Source: CAD feature listing. Evaluate the final solid. Frame: model axes, mm. Coordinates: 2 decimals unless noted, no trailing zeros. Order: outer loops, then holes, each group sorted by start corner. A loop starts at its lowest first (then second) coordinate and runs counter-clockwise, first axis right, second up. Notation, with made-up numbers: (19, 73) - (62, 73) arc R19 cw to (62, 107) - close; hole circle Ø2 at (-8, 23.5). An arc over 180 degrees is marked (long way). One line per question, with ' | ' between items.
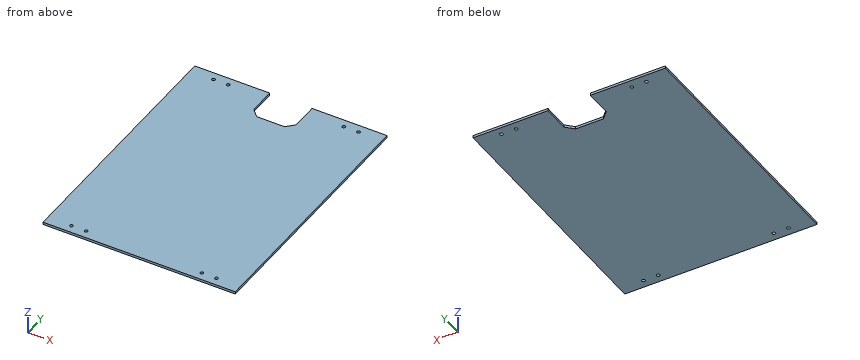
from build123d import *

# Parameters (mm, degrees)
ESQUISSE1_W             = 236
ESQUISSE1_H             = 314
BOSS_EXTRU_1_DEPTH      = 3
ENL_V_MAT_EXTRU_1_REACH = 200.829
ESQUISSE3_R             = 2
ENL_V_MAT_EXTRU_2_REACH = 200.829


with BuildPart() as part:
    # Esquisse1 → Boss.-Extru.1 (new body)
    with BuildSketch(Plane.XY):
        with Locations((0, -3)):
            Rectangle(ESQUISSE1_W, ESQUISSE1_H)
    extrude(amount=BOSS_EXTRU_1_DEPTH)

    # Esquisse3 → Enl_v. mat.-Extru.1 (cut, up to next)
    with BuildSketch(Plane.XY.offset(3), mode=Mode.PRIVATE) as enl_v_mat_extru_1_sk1:
        with Locations((-71, -150)):
            Circle(ESQUISSE3_R)
    enl_v_mat_extru_1_tool1 = extrude(enl_v_mat_extru_1_sk1.sketch, amount=-ENL_V_MAT_EXTRU_1_REACH, mode=Mode.PRIVATE) & part.part
    # Esquisse3 → Enl_v. mat.-Extru.1 (cut, up to next)
    with BuildSketch(Plane.XY.offset(3), mode=Mode.PRIVATE) as enl_v_mat_extru_1_sk2:
        with Locations((-89, -150)):
            Circle(ESQUISSE3_R)
    enl_v_mat_extru_1_tool2 = extrude(enl_v_mat_extru_1_sk2.sketch, amount=-ENL_V_MAT_EXTRU_1_REACH, mode=Mode.PRIVATE) & part.part
    # Esquisse3 → Enl_v. mat.-Extru.1 (cut, up to next)
    with BuildSketch(Plane.XY.offset(3), mode=Mode.PRIVATE) as enl_v_mat_extru_1_sk3:
        with Locations((-89, 144)):
            Circle(ESQUISSE3_R)
    enl_v_mat_extru_1_tool3 = extrude(enl_v_mat_extru_1_sk3.sketch, amount=-ENL_V_MAT_EXTRU_1_REACH, mode=Mode.PRIVATE) & part.part
    # Esquisse3 → Enl_v. mat.-Extru.1 (cut, up to next)
    with BuildSketch(Plane.XY.offset(3), mode=Mode.PRIVATE) as enl_v_mat_extru_1_sk4:
        with Locations((-71, 144)):
            Circle(ESQUISSE3_R)
    enl_v_mat_extru_1_tool4 = extrude(enl_v_mat_extru_1_sk4.sketch, amount=-ENL_V_MAT_EXTRU_1_REACH, mode=Mode.PRIVATE) & part.part
    # Esquisse3 → Enl_v. mat.-Extru.1 (cut, up to next)
    with BuildSketch(Plane.XY.offset(3), mode=Mode.PRIVATE) as enl_v_mat_extru_1_sk5:
        with Locations((71, 144)):
            Circle(ESQUISSE3_R)
    enl_v_mat_extru_1_tool5 = extrude(enl_v_mat_extru_1_sk5.sketch, amount=-ENL_V_MAT_EXTRU_1_REACH, mode=Mode.PRIVATE) & part.part
    # Esquisse3 → Enl_v. mat.-Extru.1 (cut, up to next)
    with BuildSketch(Plane.XY.offset(3), mode=Mode.PRIVATE) as enl_v_mat_extru_1_sk6:
        with Locations((89, 144)):
            Circle(ESQUISSE3_R)
    enl_v_mat_extru_1_tool6 = extrude(enl_v_mat_extru_1_sk6.sketch, amount=-ENL_V_MAT_EXTRU_1_REACH, mode=Mode.PRIVATE) & part.part
    enl_v_mat_extru_1_1 = enl_v_mat_extru_1_tool1.solids().sort_by_distance((-71, -150, 3))[0]
    add(enl_v_mat_extru_1_1, mode=Mode.SUBTRACT)
    enl_v_mat_extru_1_2 = enl_v_mat_extru_1_tool2.solids().sort_by_distance((-89, -150, 3))[0]
    add(enl_v_mat_extru_1_2, mode=Mode.SUBTRACT)
    enl_v_mat_extru_1_3 = enl_v_mat_extru_1_tool3.solids().sort_by_distance((-89, 144, 3))[0]
    add(enl_v_mat_extru_1_3, mode=Mode.SUBTRACT)
    enl_v_mat_extru_1_4 = enl_v_mat_extru_1_tool4.solids().sort_by_distance((-71, 144, 3))[0]
    add(enl_v_mat_extru_1_4, mode=Mode.SUBTRACT)
    enl_v_mat_extru_1_5 = enl_v_mat_extru_1_tool5.solids().sort_by_distance((71, 144, 3))[0]
    add(enl_v_mat_extru_1_5, mode=Mode.SUBTRACT)
    enl_v_mat_extru_1_6 = enl_v_mat_extru_1_tool6.solids().sort_by_distance((89, 144, 3))[0]
    add(enl_v_mat_extru_1_6, mode=Mode.SUBTRACT)
    enl_v_mat_extru_1 = enl_v_mat_extru_1_1 + enl_v_mat_extru_1_2 + enl_v_mat_extru_1_3 + enl_v_mat_extru_1_4 + enl_v_mat_extru_1_5 + enl_v_mat_extru_1_6  # Enl_v. mat.-Extru.1 as one shape, for the pattern or mirror that repeats it

    # Sym_trie1: Enl_v. mat.-Extru.1 across plane
    add(enl_v_mat_extru_1.mirror(Plane(origin=(0, 0, 0), x_dir=(0, 0, 1), z_dir=(1, 0, 0))), mode=Mode.SUBTRACT)

    # Esquisse5 → Enl_v. mat.-Extru.2 (cut, up to next)
    with BuildSketch(Plane.XY.offset(3), mode=Mode.PRIVATE) as enl_v_mat_extru_2_sk1:
        Polygon((0, 154), (26, 154), (26, 121), (17, 112), (-17, 112), (-26, 121), (-26, 154), align=None)
    enl_v_mat_extru_2_tool1 = extrude(enl_v_mat_extru_2_sk1.sketch, amount=-ENL_V_MAT_EXTRU_2_REACH, mode=Mode.PRIVATE) & part.part
    add(enl_v_mat_extru_2_tool1.solids().sort_by_distance((0, 133.693295, 3))[0], mode=Mode.SUBTRACT)


solid = part.part
(1) Cut plane A-A (z = 0.75). State how many separate pieces and enclosed holes the cut face has, and give its area (3 significant figures).
Taken from the geometry:
separate pieces: 1 | enclosed holes: 8 | area: 71,900 mm²
(2) Material intervals for L1, parallel to Y at x = -89, z = 1.7; L2, parallel to X at y = -150, z = 2.3; L3, parallel to Y at x = -14, z = 1.7, sorted ascending. Write a range as from..to.
Taken from the geometry:
L1: y = -160..-152, -148..142, 146..154 | L2: x = -118..-91, -87..-73, -69..69, 73..87, 91..118 | L3: y = -160..112
(3) Pin query (flat end, axial travel): P1, Ø6.5, axis at x = 89, y = 144, coming from the -Z side; P2, Ø0.9, axis at x = 2, z = 2, coming from the +Y side. Return the tip coordinate at first contact, or that it passes through.
Taken from the geometry:
P1: stops at z = 0 | P2: stops at y = 112
(4) Cut plane B-B (x = 3.5). Return the cut outline in (y, z).
Taken from the geometry:
outline: (-160, 0) - (112, 0) - (112, 3) - (-160, 3) - close
